Can you work these out from the model? Positions are in its coordinate system, mm. Face numbers are marked on the shaded views. Round coordinates to 2 decimals unless told otherwise and drop trailing zeros. Write each loop counter-clockwise with the first axis right and the second up, starting at its lowest first coordinate (ties: lowest second). Pieces come first, ordered by that corner, then holes. Notation, with made-up numbers: (33, 58.25) - (85, 58.25) arc R6 ccw to (85, 66.25) - close; hole circle Ø7 at (26, 56.25). An arc over 180 degrees is marked (long way). One line per item, written item: value. Start each with the question number.
(1) If I drill on L1, parallel to Z at x = -0.75, y = 1.5; L2, parallel to Z at x = -5, y = 7.5; L3, parallel to X at y = 3.25, z = 55, over which ranges is the centre line in solid material (lowest first)? Write a range as from..to.
(2) I want a section at C-C on y = 4. List the corners of the cut face in (x, z) for me.
(3) Thinking about a two-plate mould opening in Z: for the marked faces 1 and 2, which applies, +Z half, -Z half, draft (parallel to the pull), parting line (faces both ways), or undercut?
(4) I want a section at B-B on x = -9.75. List the corners of the cut face in (y, z) for me, plus the area to 3 significant figures.
(5) I want a section at A-A on x = -4.5. List the corners of the cut face in (y, z) for me.
(6) I want a section at D-D on z = -21.5. List the corners of the cut face in (x, y) for me, plus the area to 3 significant figures.
(7) I'm going to push flat-ended pins straight in: pin 1 Ø1 at (y, z) = (9, 28) entering from -X; pin 2 Ø3.5 at (y, z) = (7, 65.5) entering from -X; pin 3 Ø2 at (y, z) = (3, -69) entering from -X. Where does each tip first touch, or does it pass through?
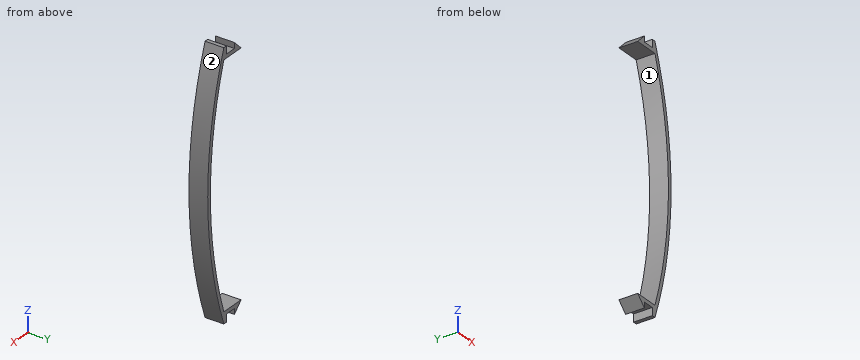
from build123d import *

# Parameters (mm, degrees)
BOSS_EXTRU_1_DEPTH = 10


with BuildPart() as part:
    # Esquisse1 → Boss.-Extru.1 (new body)
    with BuildSketch(Plane(origin=(0, 0, 0), x_dir=(1, 0, 0), z_dir=(0, 1, 0))):
        with BuildLine():
            Line((0, -61), (-13, -61))
            Line((-13, -61), (-8, -66))
            Line((-8, -66), (-8, -63))
            Line((-8, -63), (-2, -63))
            Line((-2, -63), (-2, -67.086901798))
            Line((-2, -67.086901798), (0, -67.086901798))
            ThreePointArc((0, -67.086901798), (12.181665796, 2), (0, 71.086901798))
            Line((0, 71.086901798), (-2, 71.086901798))
            Line((-2, 71.086901798), (-2, 67))
            Line((-2, 67), (-8, 67))
            Line((-8, 67), (-8, 70))
            Line((-8, 70), (-13, 65))
            Line((-13, 65), (0, 65))
            ThreePointArc((0, 65), (10.181665796, 2), (0, -61))
        make_face()
    extrude(amount=BOSS_EXTRU_1_DEPTH)


solid = part.part
Established:
1. L1: -71.09..-65, 61..67.09
1. L2: -67..-65, 61..63
1. L3: 1.89..3.97
2. outline: (-13, -65) - (-8, -70) - (-8, -67) - (-2, -67) - (-2, -71.09) - (0, -71.09) arc R202 ccw to (0, 67.09) - (-2, 67.09) - (-2, 63) - (-8, 63) - (-8, 66) - (-13, 61) - (0, 61) arc R200 cw to (0, -65) - close
3. face 1: undercut
3. face 2: parting line
4. outline: (0, -68.25) - (10, -68.25) - (10, -65) - (0, -65) - close; (0, 61) - (10, 61) - (10, 64.25) - (0, 64.25) - close
4. area: 65.0 mm2
5. outline: (0, -67) - (10, -67) - (10, -65) - (0, -65) - close; (0, 61) - (10, 61) - (10, 63) - (0, 63) - close
6. outline: (9.23, 0) - (11.24, 0) - (11.24, 10) - (9.23, 10) - close
6. area: 20.1 mm2
7. pin 1: x = 7.84
7. pin 2: x = -10.25
7. pin 3: x = -10
